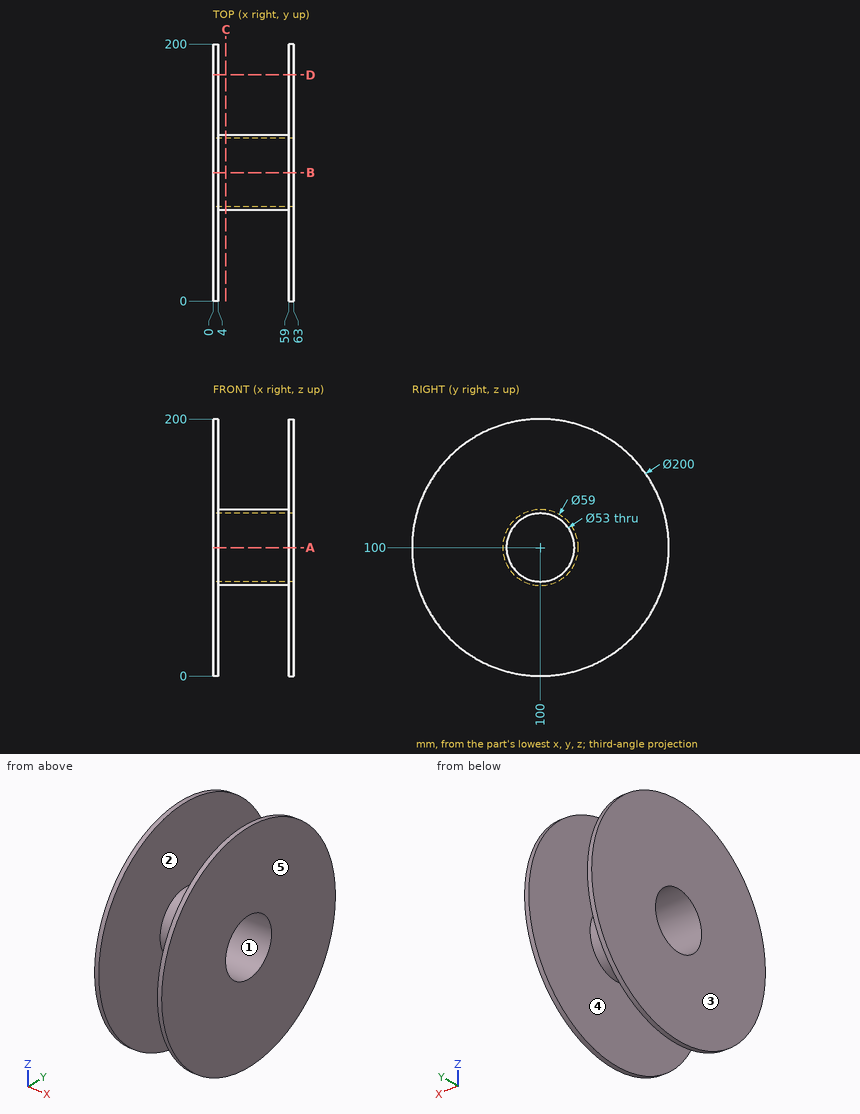
Answer from the drawing. Dimensions are ordinates in mm from the lowest x, y and z of the part. A direction names the side the tool comes from. Round coordinates to 2 decimals unless told otherwise and drop trailing zeros. Write each loop counter-clockwise with the first axis right and the second up, starting at its lowest first coordinate (ties: lowest second). Pieces come first, ordered by that corner, then holes. Notation, with made-up numbers: (-4.75, 74.5) -> (39.25, 74.5) arc R23 ccw to (39.25, 112.5) -> close; hole circle Ø4 at (71.5, 64.5). An arc over 180 degrees is marked (long way). Write each question's results on one line, items separated by ' | '.
1) The part is cut by section A-A (z = 100). Write down the section's boundary in (x, y), and give its area (3 significant figures).
Findings:
outline: (0, 0) -> (4, 0) -> (4, 70.5) -> (59, 70.5) -> (59, 0) -> (63, 0) -> (63, 73.5) -> (0, 73.5) -> close; (0, 126.5) -> (63, 126.5) -> (63, 200) -> (59, 200) -> (59, 129.5) -> (4, 129.5) -> (4, 200) -> (0, 200) -> close | area: 1,510 mm²
2) Consider line 1 along X through (y, z) = (167, 162); line 2 along Z through (x, y) = (25.5, 100); line 3 along Y through (x, z) = (37, 98.5). Determine where each line is inside the solid, lowest interval first. Write a range as [from, to].
Findings:
line 1: x = [0, 4], [59, 63] | line 2: z = [70.5, 73.5], [126.5, 129.5] | line 3: y = [70.54, 73.54], [126.46, 129.46]
3) The part is cut by section C-C (x = 10). Write down the section's boundary in (y, z).
Findings:
outline: circle Ø59 at (100, 100); hole circle Ø53 at (100, 100)
4) Flat-ended cylindrical pins translate along their axes: pin 1 (1 mm diameter, centred on y = 118, z = 24.5, fed in from -X); pin 2 (3 mm diameter, centred on x = 37, y = 113, fed in from +Z). Find the tip coordinate at first contact, or state that the pin passes through.
Findings:
pin 1: stops at x = 0 | pin 2: stops at z = 127.17
5) Which of the six approach directions +Z, -Z, +X, -X, +Y, -Y give full straight-line access (tool end or side, diameter ignored) to the marked faces 1 and 2?
Findings:
face 1: +X, -X | face 2: none
6) The part is cut by section D-D (y = 176). Write down the section's boundary in (x, z), and give its area (3 significant figures).
Findings:
outline: (0, 35.01) -> (4, 35.01) -> (4, 164.99) -> (0, 164.99) -> close; (59, 35.01) -> (63, 35.01) -> (63, 164.99) -> (59, 164.99) -> close | area: 1,040 mm²
7) For a pull along X with two mould halves and no side action, classify the marked faces 3, 4 and 5 as +X half, -X half, draft (parallel to the pull), parting line (faces both ways), or undercut.
Findings:
face 3: -X half | face 4: undercut | face 5: +X half
